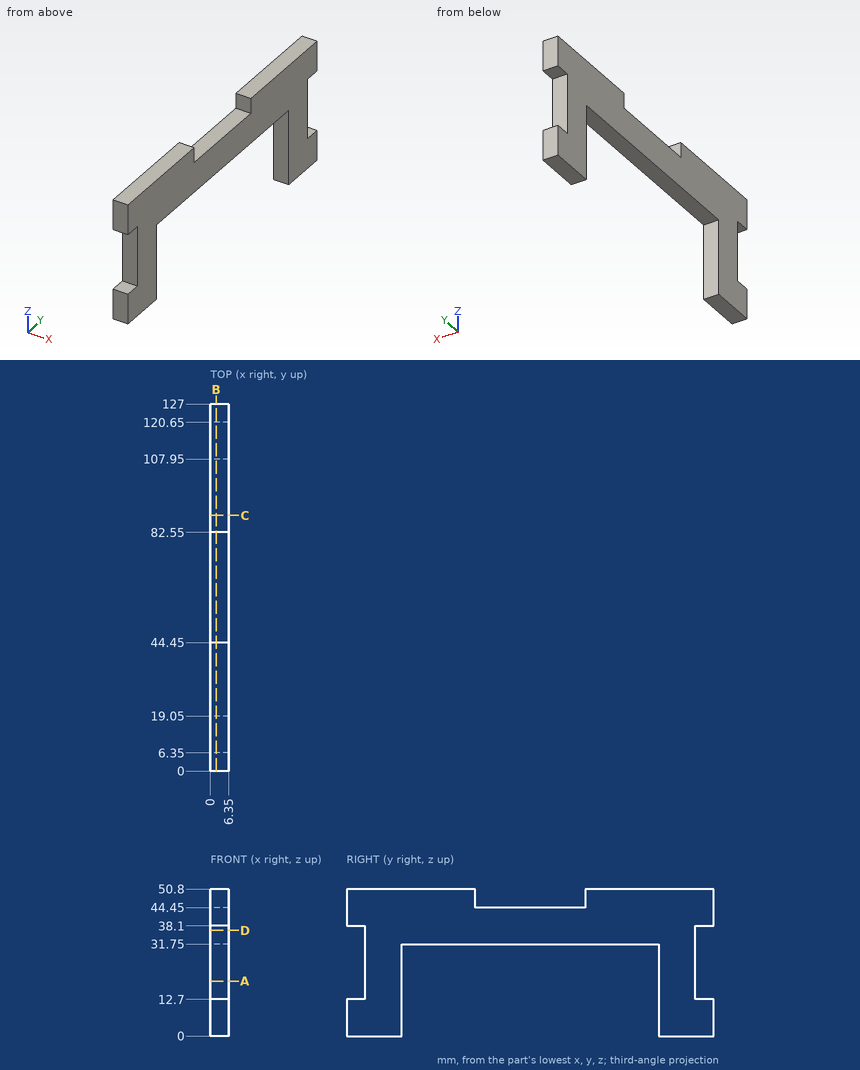
The drawing under review shows one solid part. Ordinate dimensions are in mm from its lowest x, y, z. Round coordinates to 2 decimals unless told otherwise and drop trailing zeros. Loops run counter-clockwise (first coordinate to the right, second up) from the corner with the lowest first, then second, coordinate; pieces in that order, holes last. Notation, with made-up numbers: (68.25, -19) - (119.25, -19) arc R28 ccw to (119.25, -1) - close; hole circle Ø2 at (-1.75, -25.75). An arc over 180 degrees is marked (long way). Use a Markdown table: item, result. Add a question column.
Q1. Add section B-B (x = 2). State the section outline as (y, z) points.
Q2. Add section A-A (z = 19). State the section outline as (x, y) points.
Q3. Add section D-D (z = 36.5). State the section outline as (x, y) points, plus the area to 3 significant figures.
Q4. For probe 1 along Y at (x, z) = (3, 16); probe 2 along Z at (x, y) = (1.75, 122.5); probe 3 along Y at (x, z) = (1.75, 10), list the stretches that pass through material, from the lowest coordinate up.
Q5. Insertion check: pin 1 Ø1.5 at (y, z) = (34.5, 43) entering from -X; pin 2 Ø3 at (x, y) = (1.5, 64.5) entering from -Z; pin 3 Ø1.9 at (x, y) = (4.5, 67.5) entering from +Z; pin 4 Ø1.9 at (x, z) = (3, 17.5) entering from -Y. Each pin has a flat end and moves straight along its axis. Give the tip position at first contact, or say it passes through.
Q6. Add section C-C (y = 88.5). State the section outline as (x, z) points, plus the area to 3 significant figures.
Worked answers:
| question | item | result |
|---|---|---|
| 1 | outline | (0, 0) - (19.05, 0) - (19.05, 31.75) - (107.95, 31.75) - (107.95, 0) - (127, 0) - (127, 12.7) - (120.65, 12.7) - (120.65, 38.1) - (127, 38.1) - (127, 50.8) - (82.55, 50.8) - (82.55, 44.45) - (44.45, 44.45) - (44.45, 50.8) - (0, 50.8) - (0, 38.1) - (6.35, 38.1) - (6.35, 12.7) - (0, 12.7) - close |
| 2 | outline | (0, 6.35) - (6.35, 6.35) - (6.35, 19.05) - (0, 19.05) - close; (0, 107.95) - (6.35, 107.95) - (6.35, 120.65) - (0, 120.65) - close |
| 3 | outline | (0, 6.35) - (6.35, 6.35) - (6.35, 120.65) - (0, 120.65) - close |
| 3 | area | 726 mm² |
| 4 | probe 1 | 6.35 to 19.05, 107.95 to 120.65 |
| 4 | probe 2 | 0 to 12.7, 38.1 to 50.8 |
| 4 | probe 3 | 0 to 19.05, 107.95 to 127 |
| 5 | pin 1 | x = 0 |
| 5 | pin 2 | z = 31.75 |
| 5 | pin 3 | z = 44.45 |
| 5 | pin 4 | y = 6.35 |
| 6 | outline | (0, 31.75) - (6.35, 31.75) - (6.35, 50.8) - (0, 50.8) - close |
| 6 | area | 121 mm² |
